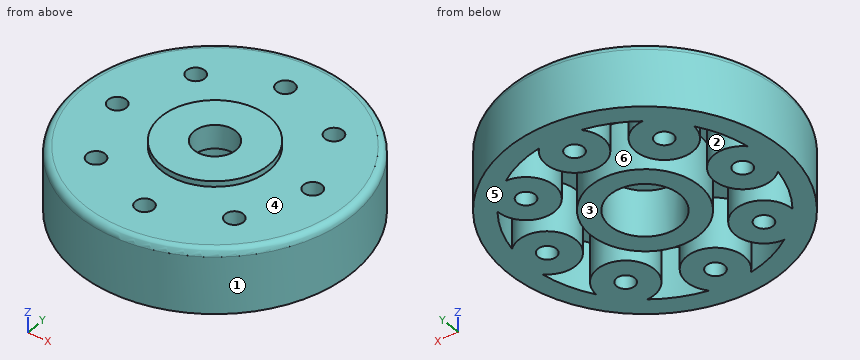
```python
from build123d import *

# Parameters (mm, degrees)
SKETCH1_R           = 9.85
SKETCH1_R_2         = 1.5
SKETCH1_R_3         = 0.65
BOSS_EXTRUDE1_DEPTH = 5
SKETCH4_R           = 2.5
CUT_EXTRUDE2_DEPTH  = 3.3
SHELL1_OUTLINE_R    = 3.9
SHELL1_DEPTH        = 3.6
CUT_EXTRUDE1_START  = -0.4
SKETCH3_R           = 9.85
SKETCH3_R_2         = 3.85
CUT_EXTRUDE1_DEPTH  = 0.4
FILLET1_R           = 0.5


# Read off the part's stored shape, not the designer's step: Shell1
with BuildPart() as part:
    # Sketch1 → Boss-Extrude1 (new body)
    with BuildSketch(Plane.XY):
        Circle(SKETCH1_R)
        Circle(SKETCH1_R_2, mode=Mode.SUBTRACT)
        with Locations((0, 6.9)):
            Circle(SKETCH1_R_3, mode=Mode.SUBTRACT)
        with Locations((4.87903679, 4.87903679)):
            Circle(SKETCH1_R_3, mode=Mode.SUBTRACT)
        with Locations((6.9, 0)):
            Circle(SKETCH1_R_3, mode=Mode.SUBTRACT)
        with Locations((4.87903679, -4.87903679)):
            Circle(SKETCH1_R_3, mode=Mode.SUBTRACT)
        with Locations((0, -6.9)):
            Circle(SKETCH1_R_3, mode=Mode.SUBTRACT)
        with Locations((-4.87903679, -4.87903679)):
            Circle(SKETCH1_R_3, mode=Mode.SUBTRACT)
        with Locations((-6.9, 0)):
            Circle(SKETCH1_R_3, mode=Mode.SUBTRACT)
        with Locations((-4.87903679, 4.87903679)):
            Circle(SKETCH1_R_3, mode=Mode.SUBTRACT)
    extrude(amount=BOSS_EXTRUDE1_DEPTH)

    # Sketch4 → Cut-Extrude2 (cut)
    with BuildSketch(Plane(origin=(0, 0, 0), x_dir=(-1, 0, 0), z_dir=(0, 0, -1))):
        Circle(SKETCH4_R)
    extrude(amount=-CUT_EXTRUDE2_DEPTH, mode=Mode.SUBTRACT)

    # Shell1 outline → Shell1 (cut)
    with BuildSketch(Plane.XY):
        with BuildLine():
            ThreePointArc((4.837035489, 6.928606474), (3.233675004, 7.80678205), (1.478964027, 8.319565217))
            ThreePointArc((1.478964027, 8.319565217), (0, 4.85), (-1.478964027, 8.319565217))
            ThreePointArc((-1.478964027, 8.319565217), (-3.233675004, 7.80678205), (-4.837035489, 6.928606474))
            ThreePointArc((-4.837035489, 6.928606474), (-3.429467889, 3.429467889), (-6.928606474, 4.837035489))
            ThreePointArc((-6.928606474, 4.837035489), (-7.80678205, 3.233675004), (-8.319565217, 1.478964027))
            ThreePointArc((-8.319565217, 1.478964027), (-4.85, 0), (-8.319565217, -1.478964027))
            ThreePointArc((-8.319565217, -1.478964027), (-7.80678205, -3.233675004), (-6.928606474, -4.837035489))
            ThreePointArc((-6.928606474, -4.837035489), (-3.429467889, -3.429467889), (-4.837035489, -6.928606474))
            ThreePointArc((-4.837035489, -6.928606474), (-3.233675004, -7.80678205), (-1.478964027, -8.319565217))
            ThreePointArc((-1.478964027, -8.319565217), (0, -4.85), (1.478964027, -8.319565217))
            ThreePointArc((1.478964027, -8.319565217), (3.233675004, -7.80678205), (4.837035489, -6.928606474))
            ThreePointArc((4.837035489, -6.928606474), (3.429467889, -3.429467889), (6.928606474, -4.837035489))
            ThreePointArc((6.928606474, -4.837035489), (7.80678205, -3.233675004), (8.319565217, -1.478964027))
            ThreePointArc((8.319565217, -1.478964027), (4.85, 0), (8.319565217, 1.478964027))
            ThreePointArc((8.319565217, 1.478964027), (7.80678205, 3.233675004), (6.928606474, 4.837035489))
            ThreePointArc((6.928606474, 4.837035489), (3.429467889, 3.429467889), (4.837035489, 6.928606474))
        make_face()
        Circle(SHELL1_OUTLINE_R, mode=Mode.SUBTRACT)
    extrude(amount=SHELL1_DEPTH, mode=Mode.SUBTRACT)

    # Sketch3 → Cut-Extrude1 (cut)
    with BuildSketch(Plane.XY.offset(5).offset(CUT_EXTRUDE1_START)):
        Circle(SKETCH3_R)
        Circle(SKETCH3_R_2, mode=Mode.SUBTRACT)
    extrude(amount=CUT_EXTRUDE1_DEPTH, mode=Mode.SUBTRACT)

    # Fillet1
    fillet1_edges = [part.edges().sort_by_distance(p)[0] for p in [
        (-9.85, 0, 4.6),
    ]]
    fillet(fillet1_edges, radius=FILLET1_R)


solid = part.part
```
Check sheet for the modelled part. Datum: model origin and axes. Units: mm. Face numbers are marked on the shaded views. A direction names the side the tool comes from. Coordinates: 2 decimals unless noted, no trailing zeros. Write item = value, one per line. Start each with the question number.
1) Access from +Z, -Z, +X, -X, +Y, -Y to the whole of each face (thin tool, end or side, straight path). Record for the marked faces 4, 5 and 6.
2) Cross-section at A-A (y = 0). State how many separate pieces and enclosed holes the cut face has, then the cut area to 3 significant figures.
3) Mould release check, pull along X, two halves, no side actions. Record for the marked faces 1, 2 and 3: +X half, -X half, draft (parallel to the pull), parting line (faces both ways), or undercut.
4) Material ranges on L1, parallel to X at y = -2.75, z = 0.45; L2, parallel to X at y = 4.5, z = 0.5; L3, parallel to X at y = -1.25, z = 1, recorded low to high.
5) Go/stop test with flat-tipped pins: P1, Ø1.5, axis at x = 6, z = 3, coming from the +Y side; P2, Ø3, axis at y = -3, z = 1, coming from the -X side; P3, Ø1, axis at x = 4.88, y = -4.88, coming from the +Z side; P4, Ø1, axis at y = 4, z = 4, coming from the +X side. Record where each tip stops, or that it passes through.
Ans:
q1.face_4 = +Z
q1.face_5 = -Z, +X, -X, +Y, -Y
q1.face_6 = -Z
q2.separate_pieces = 4
q2.enclosed_holes = 0
q2.area = 53.2 mm²
q3.face_1 = parting line
q3.face_2 = undercut
q3.face_3 = draft
q4.L1 = -9.46 to -7.99, -2.77 to 2.77, 7.99 to 9.46
q4.L2 = -8.76 to -7.15, -6.89 to -5.41, -4.35 to -2.86, 2.86 to 4.35, 5.41 to 6.89, 7.15 to 8.76
q4.L3 = -9.77 to -5.28, -3.69 to -2.17, 2.17 to 3.69, 5.28 to 9.77
q5.P1 = 8.33
q5.P2 = -9.74
q5.P3 = through
q5.P4 = 9.21
